from build123d import *

# Parameters (mm, degrees)
SKETCH3_R               = 68
BOSS_EXTRUDE1_DEPTH     = 300
SHELL1_T                = -5
CUT_EXTRUDE3_DEPTH      = 316.036505821
CUT_EXTRUDE3_DEPTH_BACK = 316.036505821


with BuildPart() as part:
    # Sketch3 → Boss-Extrude1 (new body)
    with BuildSketch(Plane(origin=(0, 0, 0), x_dir=(1, 0, 0), z_dir=(0, 1, 0))):
        with Locations(Location((0, 0, 0), (0, 0, 270))):
            Circle(SKETCH3_R)
    extrude(amount=BOSS_EXTRUDE1_DEPTH)

    # Shell1
    shell1_openings = [part.faces().sort_by_distance(p)[0] for p in [
        (0, 0, 0),
    ]]
    offset(amount=SHELL1_T, openings=shell1_openings, kind=Kind.INTERSECTION)

    # Sketch8 → Cut-Extrude3 (cut, two sides: drawn at the far end of the back side and taken through both)
    with BuildSketch(Plane.XY.offset(-CUT_EXTRUDE3_DEPTH_BACK)):
        Polygon((-68, 0), (-58, 0), (-58, 40), (-68, 50), align=None)
        Polygon((68, 0), (58, 0), (58, 40), (68, 50), align=None)
    extrude(amount=CUT_EXTRUDE3_DEPTH + CUT_EXTRUDE3_DEPTH_BACK, mode=Mode.SUBTRACT)


solid = part.part
Build history of the part. All positions in model axes, mm. A direction names the side the tool comes from. Give positions to 0.01 mm unless a question says otherwise; leave off trailing zeros. Write each loop counter-clockwise with the first axis right and the second up, starting at its lowest first coordinate (ties: lowest second). Pieces come first, ordered by that corner, then holes. Notation, with made-up numbers: (76, 57.5) - (115, 57.5) arc R16 cw to (115, 62.5) - close; hole circle Ø3 at (-25.75, -23.5). An arc over 180 degrees is marked (long way). Use one line per item in the form item = value. Start each with the question number.
1. Band-saw the part on D-D on z = 28.5. Write the cut outline in (x, y), plus the area to 3 significant figures.
2. Band-saw the part on B-B on x = 0. Write the cut outline in (y, z), plus the area to 3 significant figures.
3. Two-plate mould, pull along X, no slides. Class faces 5 (the face through (0, 0, -64)), 6 (the face through (64, 46, 0)), 7 (the face through (18.9, 145.4, 60.1)): released by +X, released by -X, zero draft, split by the parting line, or undercut.
4. 3-axis set-ups, long thin cutter, end or side, ignore diameter. For faces 1 (the face through (1, 300, -1)), 2 (the face through (1, 295, -1)), 3 (the face through (-58, 20, -30)), 4 (the face through (58, 20, -30)): which of +Z, -Z, +X, -X, +Y, -Y reach the whole face in a straight line?
5. Band-saw the part on C-C on y = 79. Write the cut outline in (x, z).
6. Band-saw the part on A-A on z = 0. Write the cut outline in (x, y), plus the area to 4 significant figures.
7. Drop flat-ended pins along their axis: pin 1 Ø5.5 at (y, z) = (21, 30.5) entering from +X; pin 2 Ø3.5 at (y, z) = (27.5, -30.5) entering from -X; pin 3 Ø8 at (x, y) = (16.5, 95) entering from +Z; pin 4 Ø5 at (x, z) = (41.5, -52) entering from -Y. Give the stop position or say it passes through.
8. Probe line 1 (X direction, y = 68.5, z = 0); line 2 (Y direction, x = 29, z = 52.5). List the from-to ranges inside material, lowest first. Write a range as [from, to].
Conclusion:
q1.outline = (-61.74, 43.74) - (-58, 40) - (-58, 0) - (-56.18, 0) - (-56.18, 295) - (56.18, 295) - (56.18, 0) - (58, 0) - (58, 40) - (61.74, 43.74) - (61.74, 300) - (-61.74, 300) - close
q1.area = 3,580 mm²
q2.outline = (0, -68) - (300, -68) - (300, 68) - (0, 68) - (0, 63) - (295, 63) - (295, -63) - (0, -63) - close
q2.area = 3,630 mm²
q3.face_5 = zero draft
q3.face_6 = released by +X
q3.face_7 = undercut
q4.face_1 = +Z, -Z, +X, -X, +Y
q4.face_2 = -Y
q4.face_3 = +Z, -Z, -X, -Y
q4.face_4 = +Z, -Z, +X, -Y
q5.outline = circle Ø136 at (0, 0); hole circle Ø126 at (0, 0)
q6.outline = (-68, 50) - (-63, 45) - (-63, 295) - (63, 295) - (63, 45) - (68, 50) - (68, 300) - (-68, 300) - close
q6.area = 3,155 mm²
q7.pin_1 = 58
q7.pin_2 = -58
q7.pin_3 = 66.84
q7.pin_4 = 0
q8.line_1 = [-68, -63], [63, 68]
q8.line_2 = [295, 300]
